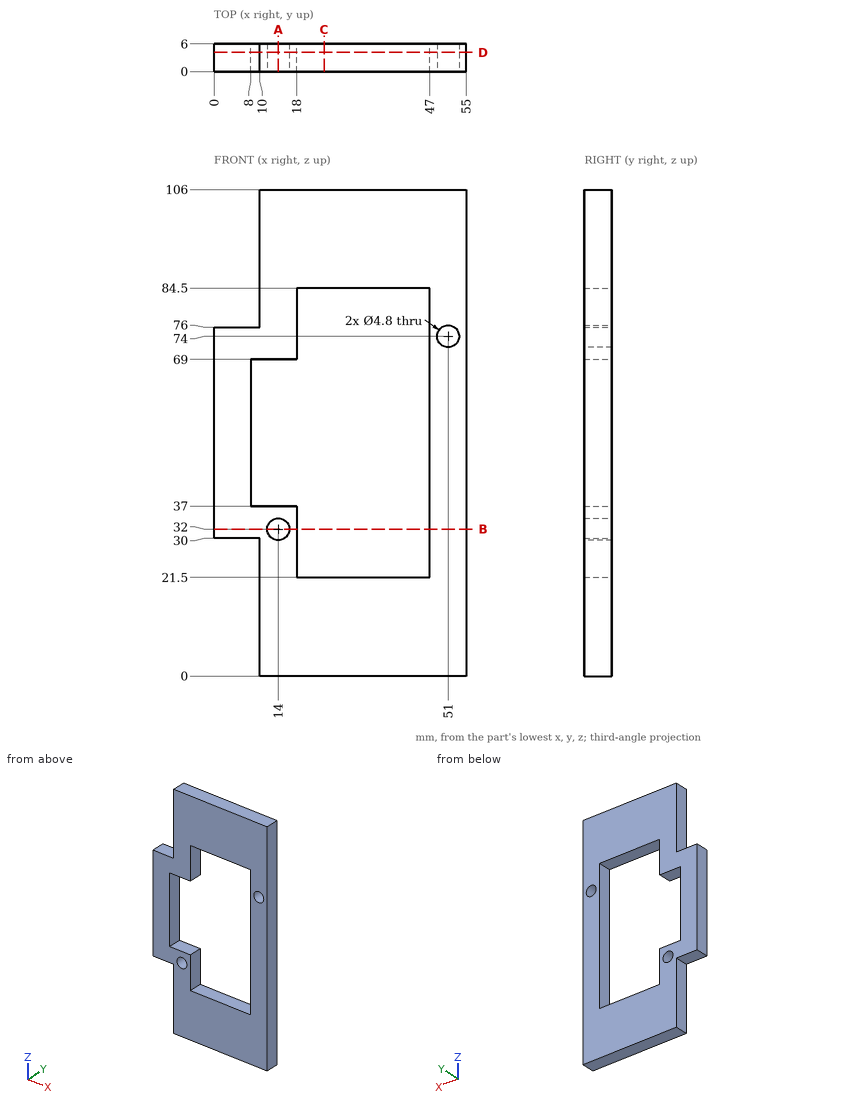
Part print with two shaded views. Sizes in mm from the minimum x, y, z corner. Coordinates: 2 decimals unless noted, no trailing zeros. Loops run counter-clockwise (first coordinate to the right, second up) from the corner with the lowest first, then second, coordinate; pieces in that order, holes last. Notation, with made-up numbers: M 0,4 L 58,4 A15 ccw 58,29 Z; hole C 2,86.25 d6. An arc over 180 degrees is marked long. Use CSV: the item, a comma, the result in double quotes. Start each with the question number.
1. Band-saw the part on A-A, the plane x = 14. List the corners of the cut face in (y, z).
2. Flat gauge pins, fed straight in: pin 1 (1.8 mm diameter, centred on y = 2, z = 89.5, fed in from -X); pin 2 (2 mm diameter, centred on x = 8.5, y = 3, fed in from +Z); pin 3 (3 mm diameter, centred on x = 5.5, y = 4.5, fed in from -Z). Where does each tip first touch, or does it go through?
3. Band-saw the part on B-B, the plane z = 32. List the corners of the cut face in (x, y).
4. Probe probe 1 along X at (y, z) = (4.1, 74); probe 2 along X at (y, z) = (1.5, 32); probe 3 along Z at (x, y) = (39.5, 3.05). List the from-to ranges inside material, lowest first. Write a range as [from, to].
5. Band-saw the part on C-C, the plane x = 24. List the corners of the cut face in (y, z), then the cut area to 3 significant figures.
6. Band-saw the part on D-D, the plane y = 4.2. List the corners of the cut face in (x, z).
Entries:
1,outline,"M 0,0 L 6,0 L 6,29.6 L 0,29.6 Z; M 0,34.4 L 6,34.4 L 6,37 L 0,37 Z; M 0,69 L 6,69 L 6,106 L 0,106 Z"
2,pin 1,"stops at x = 10"
2,pin 2,"stops at z = 76"
2,pin 3,"stops at z = 30"
3,outline,"M 0,0 L 11.6,0 L 11.6,6 L 0,6 Z; M 16.4,0 L 18,0 L 18,6 L 16.4,6 Z; M 47,0 L 55,0 L 55,6 L 47,6 Z"
4,probe 1,"x = [0, 18], [47, 48.6], [53.4, 55]"
4,probe 2,"x = [0, 11.6], [16.4, 18], [47, 55]"
4,probe 3,"z = [0, 21.5], [84.5, 106]"
5,outline,"M 0,0 L 6,0 L 6,21.5 L 0,21.5 Z; M 0,84.5 L 6,84.5 L 6,106 L 0,106 Z"
5,area,"258 mm2"
6,outline,"M 0,30 L 10,30 L 10,0 L 55,0 L 55,106 L 10,106 L 10,76 L 0,76 Z; hole M 8,37 L 18,37 L 18,21.5 L 47,21.5 L 47,84.5 L 18,84.5 L 18,69 L 8,69 Z; hole C 14,32 d4.8; hole C 51,74 d4.8"
